Print and shaded views of the part. All mm, measured from the part's lowest x, y and z. A direction names the side the tool comes from. Round coordinates to 2 decimals unless told otherwise and drop trailing zeros. Write each loop counter-clockwise with the first axis right and the second up, starting at its lowest first coordinate (ties: lowest second). Pieces come first, ordered by that corner, then holes. Notation, with made-up numbers: (13.5, 20.5) - (53.5, 20.5) arc R21 ccw to (53.5, 32.5) - close; hole circle Ø5 at (-28, -23). An arc over 180 degrees is marked (long way). One line per item, written item: value.
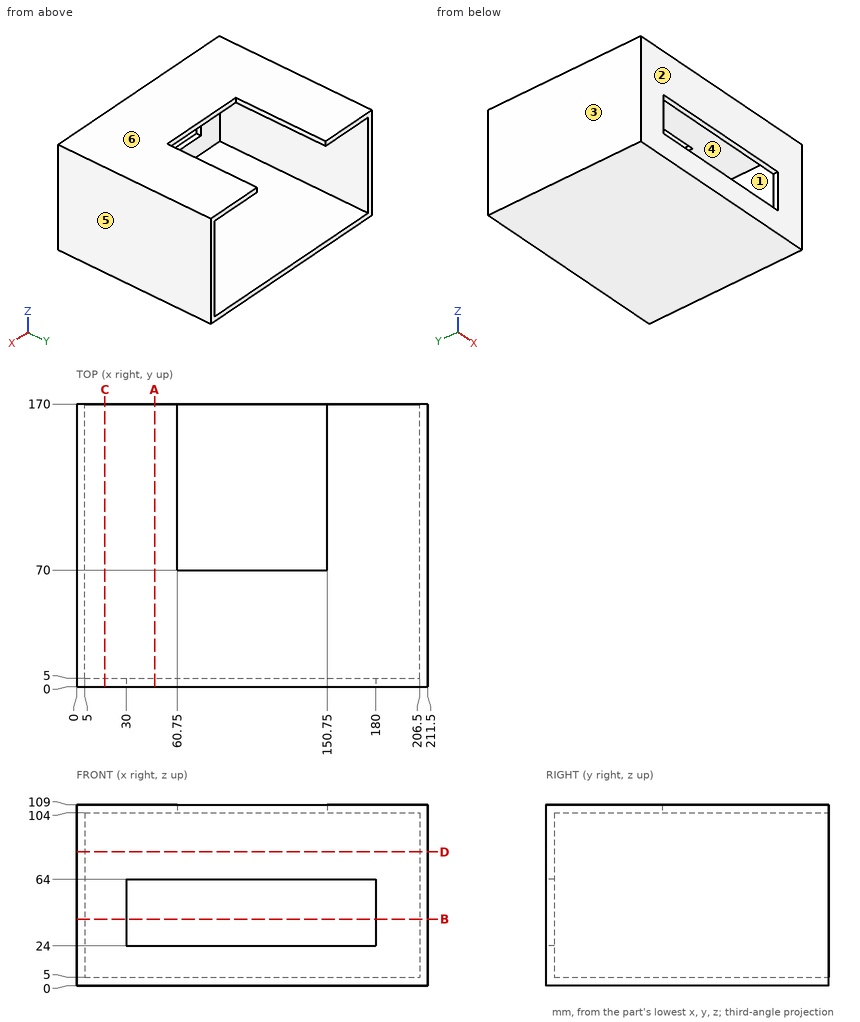
1. Wall check: probe 1 along Z at (x, y) = (34.5, 90); probe 2 along X at (y, z) = (32, 75); probe 3 along Y at (x, z) = (84, 16.5). Give the ranges that are in metal, low to high. Write a range as [from, to].
Report:
probe 1: [0, 5], [104, 109]
probe 2: [0, 5], [206.5, 211.5]
probe 3: [0, 5]
2. Drop flat-ended pins along their axis: pin 1 (12 mm diameter, centred on x = 105.5, z = 95, fed in from +Y); pin 2 (1.5 mm diameter, centred on x = 91.5, z = 105.5, fed in from +Y). Give the stop position or say it passes through.
Report:
pin 1: y = 5
pin 2: y = 70
3. Band-saw the part on C-C on x = 17. Write the cut outline in (y, z), plus the area to 4 significant figures.
Report:
outline: (0, 0) - (170, 0) - (170, 5) - (5, 5) - (5, 104) - (170, 104) - (170, 109) - (0, 109) - close
area: 2,195 mm²
4. Tool access for the marked faces 1 and 2: list every direction of +Z, -Z, +X, -X, +Y, -Y with a clear straight run to the whole face (end or side of a thin tool).
Report:
face 1: +Y
face 2: +Z, -Z, +X, -X, -Y
5. Mould opens along X. For the marked faces 3, 4, 5 and 6 say: released by +X, released by -X, zero draft, split by the parting line, or undercut.
Report:
face 3: released by -X
face 4: undercut
face 5: released by +X
face 6: zero draft
6. Band-saw the part on A-A on x = 47. Write the cut outline in (y, z), plus the area to 4 significant figures.
Report:
outline: (0, 0) - (170, 0) - (170, 5) - (5, 5) - (5, 24) - (0, 24) - close; (0, 64) - (5, 64) - (5, 104) - (170, 104) - (170, 109) - (0, 109) - close
area: 1,995 mm²
7. Band-saw the part on D-D on z = 80.5. Write the cut outline in (x, y).
Report:
outline: (0, 0) - (211.5, 0) - (211.5, 170) - (206.5, 170) - (206.5, 5) - (5, 5) - (5, 170) - (0, 170) - close
8. Band-saw the part on B-B on z = 40. Write the cut outline in (x, y), plus the area to 3 significant figures.
Report:
outline: (0, 0) - (30, 0) - (30, 5) - (5, 5) - (5, 170) - (0, 170) - close; (180, 0) - (211.5, 0) - (211.5, 170) - (206.5, 170) - (206.5, 5) - (180, 5) - close
area: 1,960 mm²
